Geometry: final body of the model. Coordinates: model frame, mm. Face numbers are marked on the shaded views. A direction names the side the tool comes from. Coordinates: 2 decimals unless noted, no trailing zeros. Use a Markdown table: item, result. Add a question column.
```python
from build123d import *

# Parameters (mm, degrees)
BOSS_EXTRUDE2_DEPTH     = 35.5
CUT_EXTRUDE1_DEPTH      = 17.75
CUT_EXTRUDE2_DEPTH      = 2.8
SKETCH5_W               = 2.8
SKETCH5_H               = 2.75
BOSS_EXTRUDE3_DEPTH     = 50
CUT_EXTRUDE3_DEPTH      = 15
CUT_EXTRUDE4_DEPTH      = 126.902937834
CUT_EXTRUDE4_DEPTH_BACK = 126.902937834
SKETCH12_W              = 1.496855304
SKETCH12_H              = 10
SKETCH12_W_2            = 1.571931937
CUT_EXTRUDE5_DEPTH      = 20
CUT_EXTRUDE6_DEPTH      = 1


with BuildPart() as part:
    # Sketch1 → Boss-Extrude2 (new body)
    with BuildSketch(Plane.XY):
        with BuildLine():
            Line((5.6, 35.6), (5.6, -15))
            add(Edge.make_bspline(
                [(5.6, -15), (5.6, -17.274393969), (1.604195195, -25.847964508), (2.415841027, -35.113621235), (3.409417942, -42.11611418)],
                knots=[0, 0, 0, 0, 0.227789152, 0.921500182, 0.921500182, 0.921500182, 0.921500182], degree=3))
            add(Edge.make_bspline(
                [(3.409417942, -42.11611418), (14.021423643, -91.198515752), (3.540705721, -122.805120936)],
                knots=[0, 0, 0, 1, 1, 1], degree=2))
            Line((3.540705721, -122.805120936), (-4.088116427, -120.408076375))
            add(Edge.make_bspline(
                [(5.6, 35.6), (-12.367874994, 33.521263174), (-8.7823866, -50.782642202), (5.954211422, -91.451497422), (-4.088116427, -120.408076375)],
                knots=[0, 0, 0, 0, 0.40530679, 1, 1, 1, 1], degree=3))
        make_face()
    extrude(amount=BOSS_EXTRUDE2_DEPTH)

    # Sketch3 → Cut-Extrude1 (cut, symmetric)
    with BuildSketch(Plane(origin=(0, 0, 0), x_dir=(0, 0, -1), z_dir=(1, 0, 0))):
        with BuildLine():
            Line((0, -14.98237842), (29.62736343, -14.98237842))
            Line((29.62736343, -14.98237842), (29.62736343, -131.572481325))
            Line((29.62736343, -131.572481325), (-60.547074518, -131.572481325))
            Line((-60.547074518, -131.572481325), (-60.547074518, -14.98237842))
            Line((-60.547074518, -14.98237842), (-35.5, -14.98237842))
            add(Edge.make_bspline(
                [(-35.5, -14.98237842), (-28.308780975, -49.75857776), (-24.077993602, -85.166412163), (-22.769212626, -120.408076375)],
                knots=[0, 0, 0, 0, 1, 1, 1, 1], degree=3))
            Line((-22.769212626, -120.408076375), (-12.75, -120.408076375))
            add(Edge.make_bspline(
                [(0, -14.98237842), (-7.191219025, -49.75857776), (-11.441219025, -85.166412163), (-12.75, -120.408076375)],
                knots=[0, 0, 0, 0, 1, 1, 1, 1], degree=3))
        make_face()
    extrude(amount=CUT_EXTRUDE1_DEPTH, both=True, mode=Mode.SUBTRACT)

    # Sketch4 → Cut-Extrude2 (cut)
    with BuildSketch(Plane(origin=(5.6, 0, 0), x_dir=(0, 0, -1), z_dir=(1, 0, 0))):
        Polygon((-2.75, 35.6), (-32.75, 35.6), (-32.75, -15.000000007), (-32.75, -32.018147114), (-2.75, -32.018147114), (-2.75, -15.000000007), align=None)
    extrude(amount=-CUT_EXTRUDE2_DEPTH, mode=Mode.SUBTRACT)

    # Sketch5 → Boss-Extrude3 (add)
    with BuildSketch(Plane(origin=(0, 35.6, 0), x_dir=(1, 0, 0), z_dir=(0, 1, 0))):
        with Locations((7, -1.375)):
            Rectangle(SKETCH5_W, SKETCH5_H)
        with Locations((7, -34.125)):
            Rectangle(SKETCH5_W, SKETCH5_H)
    extrude(amount=-BOSS_EXTRUDE3_DEPTH)

    # Sketch6 → Cut-Extrude3 (cut, symmetric)
    with BuildSketch(Plane(origin=(0, 0, 0), x_dir=(0, 0, -1), z_dir=(1, 0, 0))):
        with BuildLine():
            Line((-7.75, 34.96933844), (-14.781773193, -27.808788024))
            ThreePointArc((-14.781773193, -27.808788024), (-17.763748777, -30.474846509), (-20.744622729, -27.807556366))
            Line((-20.744622729, -27.807556366), (-27.75, 34.96933844))
            Line((-27.75, 34.96933844), (-7.75, 34.96933844))
        make_face()
    extrude(amount=CUT_EXTRUDE3_DEPTH, both=True, mode=Mode.SUBTRACT)

    # Sketch12 → Cut-Extrude4 (cut, two sides: drawn at the far end of the back side and taken through both)
    with BuildSketch(Plane(origin=(0, 0, 0), x_dir=(0, 0, -1), z_dir=(1, 0, 0)).offset(-CUT_EXTRUDE4_DEPTH_BACK)):
        with Locations((-10.144277768, -85)):
            Rectangle(SKETCH12_W, SKETCH12_H)
        with Locations((-25.408624424, -85)):
            Rectangle(SKETCH12_W_2, SKETCH12_H)
    extrude(amount=CUT_EXTRUDE4_DEPTH + CUT_EXTRUDE4_DEPTH_BACK, mode=Mode.SUBTRACT)

    # Sketch14 → Cut-Extrude5 (cut)
    with BuildSketch(Plane(origin=(0, 0, 10.89270542), x_dir=(-1, 0, 0), z_dir=(0, 0, -1))):
        Polygon((-8.720315384, -90), (6.272671273, -90), (6.272671273, -124.093634091), (-10.541100015, -124.093634091), (-10.541100015, -90), align=None)
    extrude(amount=-CUT_EXTRUDE5_DEPTH, mode=Mode.SUBTRACT)

    # Sketch15 → Cut-Extrude6 (cut)
    with BuildSketch(Plane(origin=(0, -90, 0), x_dir=(-1, 0, 0), z_dir=(0, -1, 0))):
        with BuildLine():
            Line((-5.220315384, -13.74270542), (-8.720315384, -13.74270542))
            Line((-8.720315384, -13.74270542), (-9.623354914, -13.74270542))
            Line((-9.623354914, -13.74270542), (-9.623354914, -21.74270542))
            Line((-9.623354914, -21.74270542), (-5.220315384, -21.74270542))
            ThreePointArc((-5.220315384, -21.74270542), (-1.220315384, -17.74270542), (-5.220315384, -13.74270542))
        make_face()
    extrude(amount=-CUT_EXTRUDE6_DEPTH, mode=Mode.SUBTRACT)


solid = part.part
```
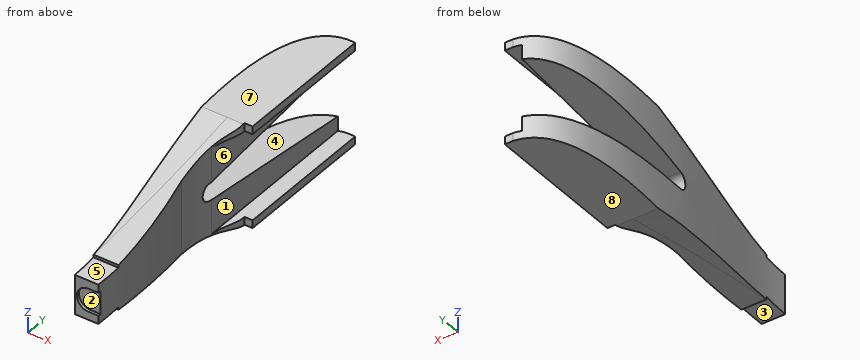
1) Draft query along Z for the marked faces 6, 7 and 8. Return one class per face: pulls with the +Z half, pulls with the -Z half, needs draft (parallel to the pull), parting line crosses it, or undercut.
2) Pin query (flat end, axial travel): pin 1 (0.5 mm diameter, centred on y = -15, z = 34, fed in from +X); pin 2 (0.5 mm diameter, centred on x = 4.5, z = 10.5, fed in from -Y); pin 3 (2.5 mm diameter, centred on x = 3.5, y = -83, fed in from +Z); pin 4 (3 mm diameter, centred on x = 4.5, y = 13, fed in from -Z). Return the tip coordinate at first contact, or that it passes through.
3) Set-up query: the marked faces 1, 2, 3, 4 and 5. Return all of +Z, -Z, +X, -X, +Y, -Y with unobstructed straight access to the full face (end or side cutting, diameter ignored); none if empty.
4) Ray query, line 1 along Z through (x, y) = (6.25, 17.5); line 2 along Z through (x, y) = (1.5, 17); line 3 along X through (y, z) = (-12.5, 24.5). Return the intervals inside material, ascending.
Values follow:
| question | item | result |
|---|---|---|
| 1 | face 6 | undercut |
| 1 | face 7 | pulls with the +Z half |
| 1 | face 8 | pulls with the -Z half |
| 2 | pin 1 | stops at x = 5.6 |
| 2 | pin 2 | stops at y = -80 |
| 2 | pin 3 | stops at z = 24.62 |
| 2 | pin 4 | stops at z = 0 |
| 3 | face 1 | +X, +Y |
| 3 | face 2 | +X, -Y |
| 3 | face 3 | -Z, +X, -X, -Y |
| 3 | face 4 | +X, -X, +Y |
| 3 | face 5 | +Z, +X, -X, -Y |
| 4 | line 1 | z = 0 to 2.75, 32.75 to 35.5 |
| 4 | line 2 | z = 0 to 9.76, 25.74 to 35.5 |
| 4 | line 3 | x = -9.13 to 2.8 |
